Input: dimensioned drawing with shaded views. Units: mm. Origin: part minimum x, y, z. A direction names the side the tool comes from. Give positions to 0.01 mm unless a question says otherwise; leave off trailing zeros. Write each loop counter-clockwise with the first axis right and the second up, starting at its lowest first coordinate (ties: lowest second). Pieces come first, ordered by that corner, then holes. Notation, with made-up numbers: (12.5, 33) -> (52.5, 33) arc R7 cw to (52.5, 40) -> close; hole circle Ø8 at (-20.5, 23.5). An arc over 180 degrees is marked (long way). Answer as a JSON object with one key per item and string values.
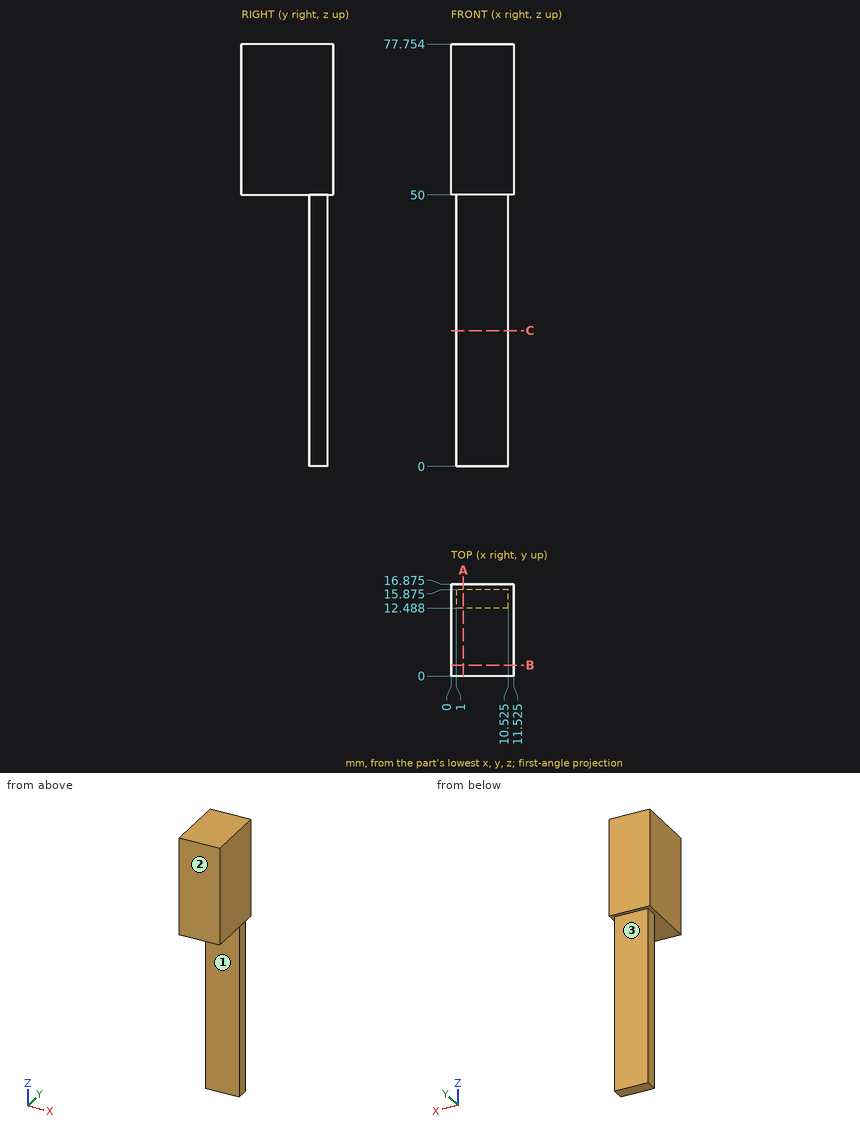
Q1. First-contact query: P1, Ø3.5, axis at y = 13.5, z = 24.5, coming from the -X side; P2, Ø2, axis at x = 5.5, z = 30, coming from the -Y side; P3, Ø3.5, axis at y = 14.5, z = 36.5, coming from the +X side (1 decimal). Flat tips, straight axial feed; report the tip coordinate or a pass-through.
Values:
{"P1": "x = 1", "P2": "y = 12.49", "P3": "x = 10.5"}
Q2. Set-up query: the marked faces 1, 2 and 3. Return all of +Z, -Z, +X, -X, +Y, -Y with unobstructed straight access to the full face (end or side cutting, diameter ignored); none if empty.
Values:
{"face 1": "-Z, +X, -X, -Y", "face 2": "+Z, -Z, +X, -X, -Y", "face 3": "-Z, +X, -X, +Y"}
Q3. Cut plane A-A (x = 2.25). Return the cut outline in (y, z) (1 decimal).
Values:
{"outline": "(0, 50) -> (12.5, 50) -> (12.5, 0) -> (15.9, 0) -> (15.9, 50) -> (16.9, 50) -> (16.9, 77.8) -> (0, 77.8) -> close"}
Q4. Cut plane C-C (z = 25). Return the cut outline in (x, y) (1 decimal).
Values:
{"outline": "(1, 12.5) -> (10.5, 12.5) -> (10.5, 15.9) -> (1, 15.9) -> close"}
Q5. Cut plane B-B (y = 2). Return the cut outline in (x, z) (1 decimal), and give its area (3 significant figures).
Values:
{"outline": "(0, 50) -> (11.5, 50) -> (11.5, 77.8) -> (0, 77.8) -> close", "area": "320 mm²"}
Q6. Material intervals for L1, parallel to X at y = 14.5, z = 36 (1 decimal); L2, parallel to Y at x = 4.5, z = 37.5 (1 decimal); L3, parallel to Z at x = 8.5, y = 2 (1 decimal), sorted ascending. Write a range as from..to.
Values:
{"L1": "1..10.5", "L2": "12.5..15.9", "L3": "50..77.8"}
